Read the model definition and answer for the solid it produces. Units are mm, in the model's axes. A direction names the side the tool comes from. Round coordinates to 2 decimals unless told otherwise and drop trailing zeros. Order: outer loops, then holes, each group sorted by start corner. A loop starts at its lowest first (then second) coordinate and runs counter-clockwise, first axis right, second up. Notation, with made-up numbers: (-10.75, 7.5) -> (35.25, 7.5) arc R10 ccw to (35.25, 13.5) -> close; hole circle Ø11 at (-3, -25). An arc over 180 degrees is marked (long way). Use a Markdown table: item, result. Add a question column.
1. Consider L1, parallel to X at y = 0.1, z = 0; L2, parallel to X at y = 0.6, z = 1; L3, parallel to Z at x = 14.5, y = 0.65. Determine where each line is inside the solid, lowest interval first. Write a range as [from, to].
2. Section A-A, the plane z = 0 is taken. Give the vertices of the cut face in (x, y).
3. Section C-C, the plane x = 18 is taken. Give the vertices of the cut face in (y, z), then the cut area to 3 significant figures.
4. Given pin 1 (1 mm diameter, centred on x = 1, y = -1, fed in from +Z); pin 2 (1.5 mm diameter, centred on x = 15.5, y = -0.5, fed in from -Z); pin 3 (1.5 mm diameter, centred on x = 2, y = -0.5, fed in from -Z); pin 4 (1 mm diameter, centred on y = 0, z = -0.5, fed in from +X), each flat-ended and moving along its own axis, determine where each tip first touches the part or whether it passes through.
5. The mould has two halves that part along Z. Classify faces 1 (the face through (9.6, 0.021, 2.247)), 2 (the face through (1, 0, -2)), 3 (the face through (18.765, -0.021, 0.806)): +Z half, -Z half, draft (parallel to the pull), parting line (faces both ways), or undercut.
6. Section B-B, the plane y = 0.95 is taken. Give the vertices of the cut face in (x, z).
7. For faces 4 (the face through (-8.999, 0.021, -2.502)), 5 (the face through (15, 0, -3)), 6 (the face through (-9.07, 0.02, 2.53)), 7 (the face through (-16.235, -0.021, 0.806)), 8 (the face through (14, 0, 3)), determine the directions among +Z, -Z, +X, -X, +Y, -Y from which every point of the face is accessible in a straight line to the end or side of a thin tool.
```python
from build123d import *

# Parameters (mm, degrees)
SKETCH1_R           = 1.5
BOSS_EXTRUDE1_DEPTH = 1.5


with BuildPart() as part:
    # Sketch1 → Boss-Extrude1 (new, symmetric)
    with BuildSketch(Plane(origin=(0, 0, 0), x_dir=(1, 0, 0), z_dir=(0, 1, 0))):
        with BuildLine():
            ThreePointArc((-17.5, 4), (-21.5, 0), (-17.5, -4))
            Line((-17.5, -4), (-11.5, -4))
            ThreePointArc((-11.5, -4), (-9.036924503, -2.516685226), (-6.208497378, -2))
            Line((-6.208497378, -2), (7.627016654, -2))
            ThreePointArc((7.627016654, -2), (9.627016654, -2.254033308), (11.5, -3))
            Line((11.5, -3), (17.5, -3))
            ThreePointArc((17.5, -3), (20.5, 0), (17.5, 3))
            Line((17.5, 3), (11.5, 3))
            ThreePointArc((11.5, 3), (9.627016654, 2.254033308), (7.627016654, 2))
            Line((7.627016654, 2), (-6.208497378, 2))
            ThreePointArc((-6.208497378, 2), (-9.036924503, 2.516685226), (-11.5, 4))
            Line((-11.5, 4), (-17.5, 4))
        make_face()
        with Locations(Location((-17.5, 0, 0), (0, 0, 270))):
            Circle(SKETCH1_R, mode=Mode.SUBTRACT)
        with Locations(Location((17.5, 0, 0), (0, 0, 270))):
            Circle(SKETCH1_R, mode=Mode.SUBTRACT)
    extrude(amount=BOSS_EXTRUDE1_DEPTH, both=True)


solid = part.part
```
Verdict:
| question | item | result |
|---|---|---|
| 1 | L1 | x = [-21.5, -19], [-16, 16], [19, 20.5] |
| 1 | L2 | x = [-21.37, -18.62], [-16.38, 16.38], [18.62, 20.33] |
| 1 | L3 | z = [-3, 3] |
| 2 | outline | (-21.5, -1.5) -> (-19, -1.5) -> (-19, 1.5) -> (-21.5, 1.5) -> close; (-16, -1.5) -> (16, -1.5) -> (16, 1.5) -> (-16, 1.5) -> close; (19, -1.5) -> (20.5, -1.5) -> (20.5, 1.5) -> (19, 1.5) -> close |
| 3 | outline | (-1.5, -2.96) -> (1.5, -2.96) -> (1.5, -1.41) -> (-1.5, -1.41) -> close; (-1.5, 1.41) -> (1.5, 1.41) -> (1.5, 2.96) -> (-1.5, 2.96) -> close |
| 3 | area | 9.26 mm2 |
| 4 | pin 1 | stops at z = 2 |
| 4 | pin 2 | stops at z = -3 |
| 4 | pin 3 | stops at z = -2 |
| 4 | pin 4 | stops at x = 20.5 |
| 5 | face 1 | +Z half |
| 5 | face 2 | -Z half |
| 5 | face 3 | undercut |
| 6 | outline | (-17.5, -4) -> (-11.5, -4) arc R8 cw to (-6.21, -2) -> (7.63, -2) arc R8 cw to (11.5, -3) -> (17.5, -3) arc R3 ccw to (17.5, 3) -> (11.5, 3) arc R8 cw to (7.63, 2) -> (-6.21, 2) arc R8 cw to (-11.5, 4) -> (-17.5, 4) arc R4 ccw to start; hole circle Ø3 at (-17.5, 0); hole circle Ø3 at (17.5, 0) |
| 7 | face 4 | -Z, +Y, -Y |
| 7 | face 5 | -Z, +X, +Y, -Y |
| 7 | face 6 | +Z, +Y, -Y |
| 7 | face 7 | +Y, -Y |
| 7 | face 8 | +Z, +X, +Y, -Y |
